Geometry check sheet. Reference: the model listing, model coordinates, mm. Face numbers are marked on the shaded views. A direction names the side the tool comes from. Round coordinates to 2 decimals unless told otherwise and drop trailing zeros. Order: outer loops, then holes, each group sorted by start corner. A loop starts at its lowest first (then second) coordinate and runs counter-clockwise, first axis right, second up. Notation, with made-up numbers: (-29, -22.5) - (24, -22.5) arc R20 ccw to (24, 15.5) - close; hole circle Ø9 at (5.25, 7). An arc over 180 degrees is marked (long way). Use a Markdown table: item, result. Add a question column.
(1) Section check B-B on x = 0. Record the boundary of the cut face in (y, z).
(2) Section check D-D on x = 6.5. Record the boundary of the cut face in (y, z).
(3) Section check C-C on z = 0. Record the boundary of the cut face in (x, y), then the cut area to 3 significant figures.
(4) Thickness scan on line 1 along Y through (x, z) = (0, 6); line 2 along X through (y, z) = (21, 7). Record the ranges inside material, lowest first. Write a range as [from, to].
(5) Access from +Z, -Z, +X, -X, +Y, -Y to the whole of each face (thin tool, end or side, straight path). Record for the marked faces 1, 2, 3 and 4.
(6) Gauge pin test, flat ends, axial feed: P1, Ø4, axis at y = 19, z = 6.5, coming from the +X side; P2, Ø6, axis at x = -3.5, y = 17.5, coming from the -Z side; P3, Ø4, axis at y = 15, z = 5.5, coming from the -X side. Record the tip position at first contact, or that the pin passes through.
(7) Section check A-A on y = 21. Record the boundary of the cut face in (x, z), then the cut area to 3 significant figures.
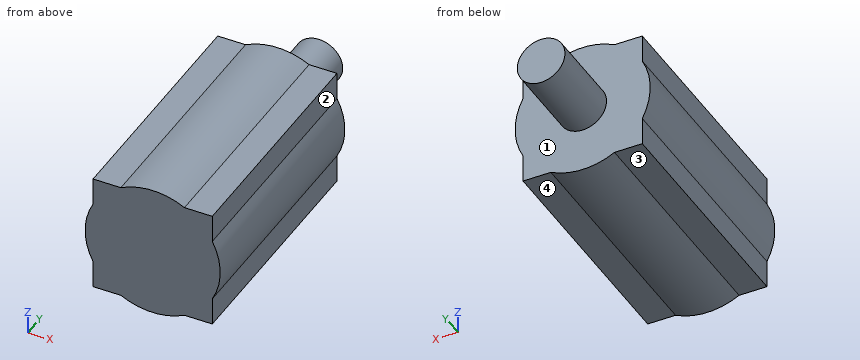
```python
from build123d import *

# Parameters (mm, degrees)
SKETCH1_R           = 8.5
SKETCH1_W           = 15
SKETCH1_H           = 15
BOSS_EXTRUDE1_DEPTH = 30
SKETCH2_R           = 3
BOSS_EXTRUDE2_DEPTH = 10


with BuildPart() as part:
    # Sketch1 → Boss-Extrude1 (new body)
    with BuildSketch(Plane(origin=(0, 0, 0), x_dir=(1, 0, 0), z_dir=(0, 1, 0))):
        Circle(SKETCH1_R)
        Rectangle(SKETCH1_W, SKETCH1_H)
    extrude(amount=BOSS_EXTRUDE1_DEPTH)

    # Sketch2 → Boss-Extrude2 (add)
    with BuildSketch(Plane(origin=(0, 30, 0), x_dir=(1, 0, 0), z_dir=(0, 1, 0))):
        with Locations(Location((0, 0, 0), (0, 0, 90))):
            Circle(SKETCH2_R)
    extrude(amount=BOSS_EXTRUDE2_DEPTH)


solid = part.part
```
Check sheet entries:
| question | item | result |
|---|---|---|
| 1 | outline | (0, -8.5) - (30, -8.5) - (30, -3) - (40, -3) - (40, 3) - (30, 3) - (30, 8.5) - (0, 8.5) - close |
| 2 | outline | (0, -7.5) - (30, -7.5) - (30, 7.5) - (0, 7.5) - close |
| 3 | outline | (-8.5, 0) - (8.5, 0) - (8.5, 30) - (3, 30) - (3, 40) - (-3, 40) - (-3, 30) - (-8.5, 30) - close |
| 3 | area | 570 mm2 |
| 4 | line 1 | y = [0, 30] |
| 4 | line 2 | x = [-7.5, 7.5] |
| 5 | face 1 | +Y |
| 5 | face 2 | +Z, +X, +Y, -Y |
| 5 | face 3 | -Z, -X, +Y, -Y |
| 5 | face 4 | -Z, +X, +Y, -Y |
| 6 | P1 | stops at x = 7.5 |
| 6 | P2 | stops at z = -8.49 |
| 6 | P3 | stops at x = -7.75 |
| 7 | outline | (-7.5, -7.5) - (-4, -7.5) arc R8.5 ccw to (4, -7.5) - (7.5, -7.5) - (7.5, -4) arc R8.5 ccw to (7.5, 4) - (7.5, 7.5) - (4, 7.5) arc R8.5 ccw to (-4, 7.5) - (-7.5, 7.5) - (-7.5, 4) arc R8.5 ccw to (-7.5, -4) - close |
| 7 | area | 247 mm2 |
